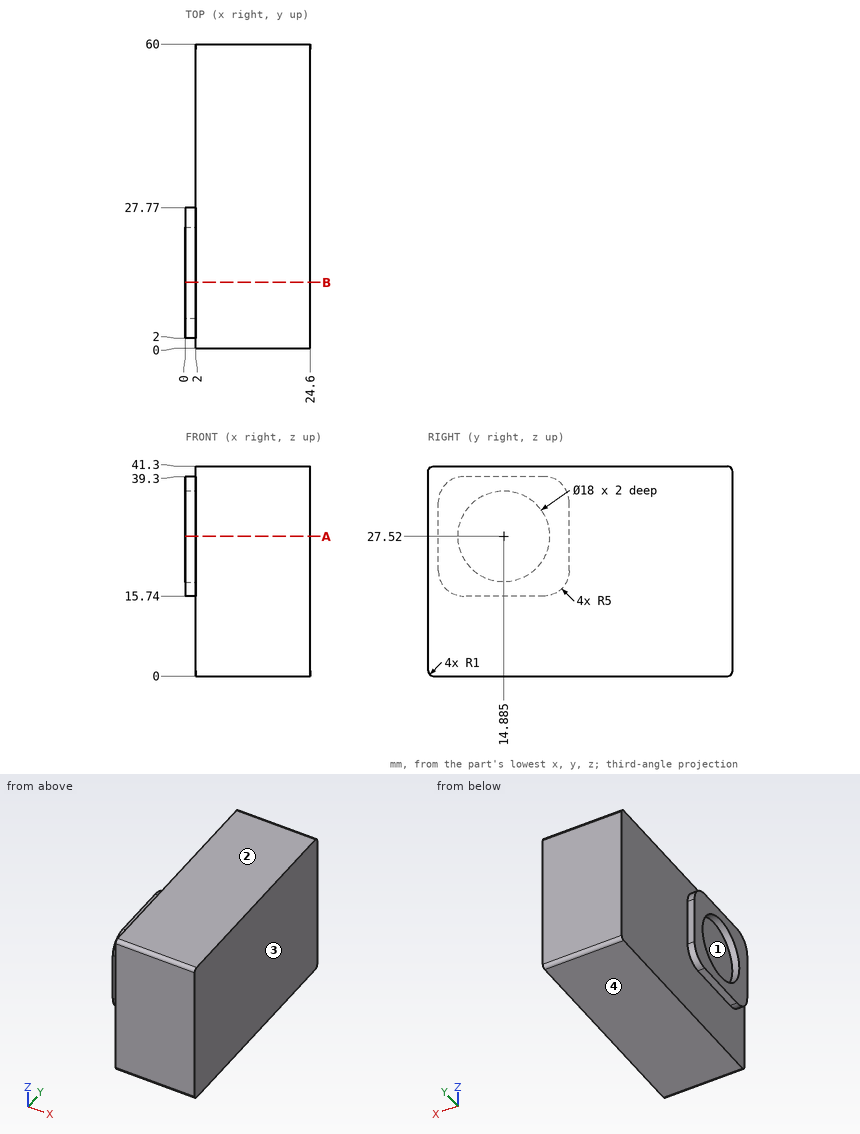
Design review of the part shown in the three views and the two pictorial views. Dimensions are in mm from the part's minimum x, y and z. Round coordinates to 2 decimals unless told otherwise and drop trailing zeros. Write each loop counter-clockwise with the first axis right and the second up, starting at its lowest first coordinate (ties: lowest second). Pieces come first, ordered by that corner, then holes. Notation, with made-up numbers: (-15.75, 46) - (26.25, 46) arc R21 ccw to (26.25, 74) - close; hole circle Ø9 at (-7.75, 38). An arc over 180 degrees is marked (long way). Write item = value, one per line. Start each with the question number.
1. Draft analysis for pull direction Z (two halves, no side actions). For the marked faces 1, 2, 3 and 4, state which applies: released by +Z, released by -Z, zero draft, split by the parting line, or undercut.
2. Consider section A-A on z = 27.52. State the section outline as (x, y) points (3 decimals), plus the area to 3 significant figures.
3. For pin 1 Ø16 at (y, z) = (14.885, 27.52) entering from -X; pin 2 Ø0.6 at (x, z) = (1, 30) entering from +Y; pin 3 Ø2 at (x, y) = (0.5, 17.5) entering from +Z, all flat-tipped, find the tip position at first contact; note any pin that passes through.
4. Wall thickness on L1, parallel to X at y = 34, z = 28.5: over which ranges is the line inside the solid? List them lowest first.
5. Consider section B-B on y = 13. State the section outline as (x, z) points, plus the area to 3 significant figures.
Evaluation:
q1.face_1 = undercut
q1.face_2 = released by +Z
q1.face_3 = zero draft
q1.face_4 = released by -Z
q2.outline = (0, 2) - (2, 2) - (2, 0) - (24.6, 0) - (24.6, 60) - (2, 60) - (2, 27.77) - (0, 27.77) - (0, 23.885) - (2, 23.885) - (2, 5.885) - (0, 5.885) - close
q2.area = 1,370 mm2
q3.pin_1 = 2
q3.pin_2 = 27.77
q3.pin_3 = 39.3
q4.L1 = 2 to 24.6
q5.outline = (0, 15.74) - (2, 15.74) - (2, 0) - (24.6, 0) - (24.6, 41.3) - (2, 41.3) - (2, 39.3) - (0, 39.3) - (0, 36.32) - (2, 36.32) - (2, 18.72) - (0, 18.72) - close
q5.area = 945 mm2
